from build123d import *

# Parameters (mm, degrees)
ESQUISSE1_R        = 3.5
ESQUISSE1_R_2      = 2
BOSS_EXTRU_2_DEPTH = 19
BOSS_EXTRU_3_START = 6
ESQUISSE1_4_R      = 2
BOSS_EXTRU_3_DEPTH = 4
BOSS_EXTRU_4_START = 15
ESQUISSE1_5_R      = 2
BOSS_EXTRU_4_DEPTH = 4


with BuildPart() as part:
    # Esquisse1 → Boss.-Extru.2 (new body)
    with BuildSketch(Plane.XY):
        Circle(ESQUISSE1_R)
        Circle(ESQUISSE1_R_2, mode=Mode.SUBTRACT)
        with BuildLine():
            Line((10.444878499, 5.315154571), (-0.583333333, 3.45104654))
            ThreePointArc((-0.583333333, 3.45104654), (2.259240285, 2.673169155), (3.5, 0))
            ThreePointArc((3.5, 0), (2.259240285, -2.673169155), (-0.583333333, -3.45104654))
            Line((-0.583333333, -3.45104654), (10.444878499, -5.315154571))
            ThreePointArc((10.444878499, -5.315154571), (8, 0), (10.444878499, 5.315154571))
        make_face()
    extrude(amount=BOSS_EXTRU_2_DEPTH)

    # Esquisse1_4 → Boss.-Extru.3 (add)
    with BuildSketch(Plane.XY.offset(BOSS_EXTRU_3_START)):
        with BuildLine():
            Line((14, 5.916079783), (10.444878499, 5.315154571))
            ThreePointArc((10.444878499, 5.315154571), (8, 0), (10.444878499, -5.315154571))
            Line((10.444878499, -5.315154571), (14, -5.916079783))
            ThreePointArc((14, -5.916079783), (21, 0), (14, 5.916079783))
        make_face()
        with Locations((15, 0)):
            Circle(ESQUISSE1_4_R, mode=Mode.SUBTRACT)
    extrude(amount=BOSS_EXTRU_3_DEPTH)

    # Esquisse1_5 → Boss.-Extru.4 (add)
    with BuildSketch(Plane.XY.offset(BOSS_EXTRU_4_START)):
        with BuildLine():
            Line((14, 5.916079783), (10.444878499, 5.315154571))
            ThreePointArc((10.444878499, 5.315154571), (8, 0), (10.444878499, -5.315154571))
            Line((10.444878499, -5.315154571), (14, -5.916079783))
            ThreePointArc((14, -5.916079783), (21, 0), (14, 5.916079783))
        make_face()
        with Locations((15, 0)):
            Circle(ESQUISSE1_5_R, mode=Mode.SUBTRACT)
    extrude(amount=BOSS_EXTRU_4_DEPTH)


solid = part.part
Geometry: final body of the model. Coordinates: model frame, mm. A direction names the side the tool comes from. Give positions to 0.01 mm unless a question says otherwise; leave off trailing zeros. Loops run counter-clockwise (first coordinate to the right, second up) from the corner with the lowest first, then second, coordinate; pieces in that order, holes last. Notation, with made-up numbers: M 38,-27.5 L 69,-27.5 A13 ccw 69,-9.5 Z; hole C -11.5,18 d7. An arc over 180 degrees is marked long. Put each result on its own line as item: value.
1) Reachability of faces 4 (the flat face through (5, 0, 0)), 5 (the cylindrical face through (8, 0, 3)), 6 (the cylindrical face through (8, 0, 12)) from +Z, -Z, +X, -X, +Y, -Y: full face, straight path, thin tool, end or side. Return the list, or none.
Computed values:
face 4: -Z, +X, -X, +Y, -Y
face 5: -Z, +X
face 6: +X
2) Cut plane D-D, the plane z = 4. Return the cut outline in (x, y), plus the area to 3 significant figures.
Computed values:
outline: M -0.58,-3.45 L 10.44,-5.32 A7 cw 10.44,5.32 L -0.58,3.45 A3.5 ccw Z; hole C 0,0 d4
area: 81.2 mm^2
3) Mould query, pull axis Y, two halves, no side actions, for faces 1 (the cylindrical face through (21, 0, 17)), 2 (the flat face through (11, 0, 19)), 3 (the flat face through (13, 1, 6)). Classes: released by +Y, released by -Y, zero draft, split by the parting line, or undercut.
Computed values:
face 1: split by the parting line
face 2: zero draft
face 3: undercut
4) Cut plane C-C, the plane x = 0. Return the cut outline in (y, z).
Computed values:
outline: M -3.55,0 L -2,0 L -2,19 L -3.55,19 Z; M 2,0 L 3.55,0 L 3.55,19 L 2,19 Z
5) Cut plane A-A, the plane y = 0. Return the cut outline in (x, z).
Computed values:
outline: M -3.5,0 L -2,0 L -2,19 L -3.5,19 Z; M 2,0 L 8,0 L 8,6 L 13,6 L 13,10 L 8,10 L 8,15 L 13,15 L 13,19 L 2,19 Z; M 17,6 L 21,6 L 21,10 L 17,10 Z; M 17,15 L 21,15 L 21,19 L 17,19 Z
6) Material intervals for L1, parallel to Z at x = 9.5, y = -1.5; L2, parallel to Y at x = 15, z = 8.3; L3, parallel to X at y = -1.5, z = 16.25, sorted ascending. Write a range as from..to.
Computed values:
L1: z = 6..10, 15..19
L2: y = -6..-2, 2..6
L3: x = -3.16..-1.32, 1.32..13.68, 16.32..20.81
7) Cut plane B-B, the plane x = 15. Return the cut outline in (y, z).
Computed values:
outline: M -6,6 L -2,6 L -2,10 L -6,10 Z; M -6,15 L -2,15 L -2,19 L -6,19 Z; M 2,6 L 6,6 L 6,10 L 2,10 Z; M 2,15 L 6,15 L 6,19 L 2,19 Z
8) First-contact query: P1, Ø3, axis at x = 6.5, z = 7.5, coming from the -Y side; P2, Ø4, axis at x = 16, y = -1.5, coming from the -Z side; P3, Ø1.5, axis at x = 11, z = 10, coming from the -Y side. Flat tips, straight axial feed; report the tip coordinate or a pass-through.
Computed values:
P1: stops at y = -4.9
P2: stops at z = 6
P3: stops at y = -5.54
